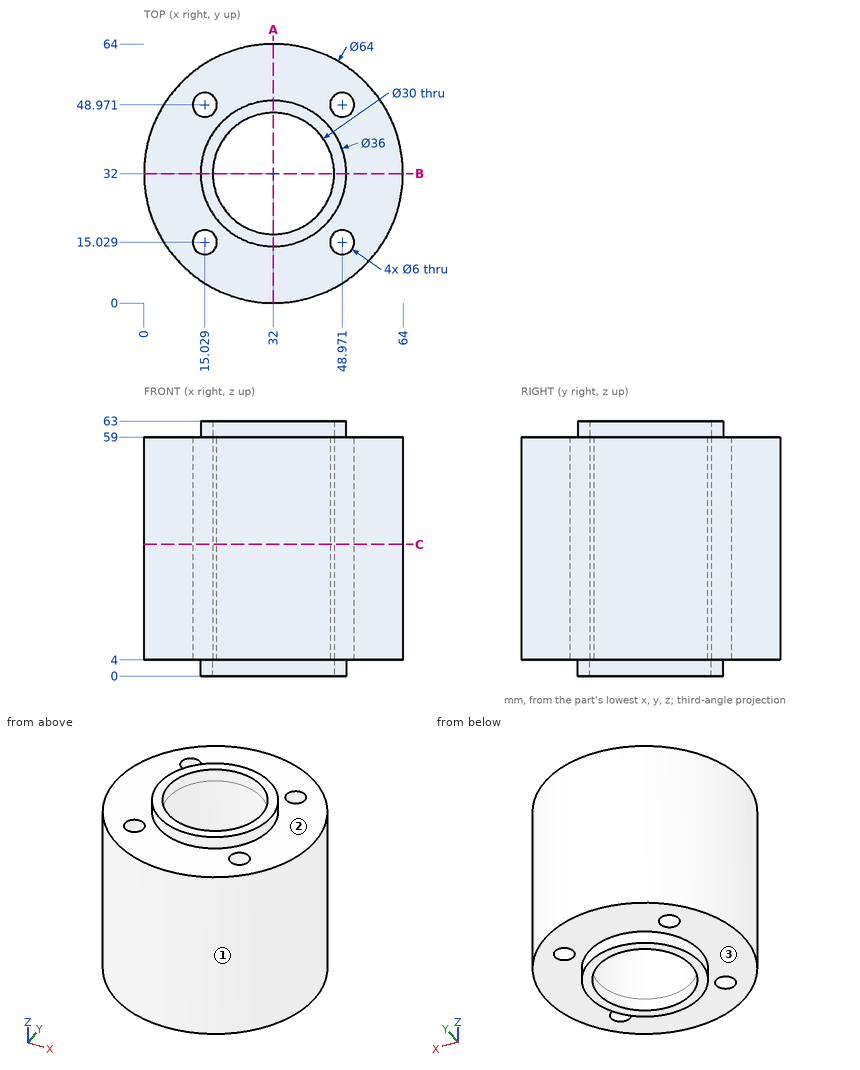
The figure shows three views and two pictorial views of one solid part (mm, origin at its lowest corner). Answer the questions. A direction names the side the tool comes from. Give positions to 0.01 mm unless a question says otherwise; leave off trailing zeros. Write each loop counter-clockwise with the first axis right and the second up, starting at its lowest first coordinate (ties: lowest second). Pieces come first, ordered by that corner, then holes. Notation, with made-up numbers: M 63,-38.75 L 78,-38.75 A11 cw 78,-25.75 Z; hole C 69,19.5 d1. An arc over 180 degrees is marked long. One line per item, written item: value. Start each with the question number.
(1) Find section C-C (z = 32.5). Determine the outline of the cut face in (x, y).
(2) Flat-ended cylindrical pins translate along their axes: pin 1 Ø10 at (x, z) = (7.5, 19) entering from +Y; pin 2 Ø6 at (x, z) = (20.5, 53) entering from +Y; pin 3 Ø9.5 at (x, y) = (15.03, 48.97) entering from +Z; pin 4 Ø18 at (x, y) = (32, 32) entering from -Z. Find the tip coordinate at first contact, or state that the pin passes through.
(3) A tool of negligible diameter and unlimited length cuts with its end or side. For the marked faces 1, 2 and 3, from which of +Z, -Z, +X, -X, +Y, -Y can it reach the whole face along a straight path? Write none if from no direction.
(4) Find the intervals of material crossed by line 1 (Y direction, x = 32, z = 61); line 2 (X direction, y = 51, z = 42); line 3 (Y direction, x = 14, z = 13), in increasing order.
(5) Find section A-A (x = 32). Determine the outline of the cut face in (y, z), plus the area to 3 significant figures.
Results below:
1. outline: C 32,32 d64; hole C 15.03,15.03 d6; hole C 15.03,48.97 d6; hole C 32,32 d30; hole C 48.97,15.03 d6; hole C 48.97,48.97 d6
2. pin 1: stops at y = 57.37
2. pin 2: stops at y = 62.85
2. pin 3: stops at z = 59
2. pin 4: passes through
3. face 1: +Z, -Z
3. face 2: +Z
3. face 3: -Z
4. line 1: y = 14 to 17, 47 to 50
4. line 2: x = 6.25 to 12.82, 17.24 to 46.76, 51.18 to 57.75
4. line 3: y = 5.54 to 12.21, 17.85 to 46.15, 51.79 to 58.46
5. outline: M 0,4 L 14,4 L 14,0 L 17,0 L 17,63 L 14,63 L 14,59 L 0,59 Z; M 47,0 L 50,0 L 50,4 L 64,4 L 64,59 L 50,59 L 50,63 L 47,63 Z
5. area: 1,920 mm^2
